```python
from build123d import *

# Parameters (mm, degrees)
BOSS_EXTRUDE1_DEPTH = 6.35
BOSS_EXTRUDE2_DEPTH = 6.604
SKETCH3_W           = 53.34
SKETCH3_H           = 69.85
BOSS_EXTRUDE3_DEPTH = 38.185673152
FILLET1_R           = 2.54
SKETCH4_W           = 25.4
SKETCH4_H           = 25.4
CUT_EXTRUDE1_DEPTH  = 70.358
CUT_EXTRUDE2_DEPTH  = 89.255701154


with BuildPart() as part:
    # Sketch1 → Boss-Extrude1 (new body)
    with BuildSketch(Plane(origin=(0, 0, 0), x_dir=(1, 0, 0), z_dir=(0, 1, 0))):
        with BuildLine():
            Line((-12.7, 0), (-12.7, 25.4))
            ThreePointArc((-12.7, 25.4), (0, 38.1), (12.7, 25.4))
            Line((12.7, 25.4), (12.7, 0))
            ThreePointArc((12.7, 0), (0, -12.7), (-12.7, 0))
        make_face()
    extrude(amount=BOSS_EXTRUDE1_DEPTH)

    # Sketch2 → Boss-Extrude2 (add)
    with BuildSketch(Plane(origin=(0, 6.35, 0), x_dir=(1, 0, 0), z_dir=(0, 1, 0))):
        with BuildLine():
            Line((-6.35, 0), (-6.35, 25.4))
            ThreePointArc((-6.35, 25.4), (0, 31.75), (6.35, 25.4))
            Line((6.35, 25.4), (6.35, 0))
            ThreePointArc((6.35, 0), (0, -6.35), (-6.35, 0))
        make_face()
    extrude(amount=BOSS_EXTRUDE2_DEPTH)

    # Sketch3 → Boss-Extrude3 (add)
    with BuildSketch(Plane(origin=(0, 12.954, 0), x_dir=(1, 0, 0), z_dir=(0, 1, 0))):
        with Locations((0.81256739, 13.33105678)):
            Rectangle(SKETCH3_W, SKETCH3_H)
    extrude(amount=BOSS_EXTRUDE3_DEPTH)

    # Fillet1
    fillet1_edges = [part.edges().sort_by_distance(p)[0] for p in [
        (-12.7, 0, -12.7),
        (0, 0, -38.1),
        (12.7, 0, -12.7),
        (0, 0, 12.7),
    ]]
    fillet(fillet1_edges, radius=FILLET1_R)

    # Sketch4 → Cut-Extrude1 (cut)
    with BuildSketch(Plane(origin=(0, 0, -48.25605678), x_dir=(-1, 0, 0), z_dir=(0, 0, -1))):
        with Locations((0, 38.439673152)):
            Rectangle(SKETCH4_W, SKETCH4_H)
    extrude(amount=-CUT_EXTRUDE1_DEPTH, mode=Mode.SUBTRACT)

    # Sketch5 → Cut-Extrude2 (cut, through all)
    with BuildSketch(Plane(origin=(27.48256739, 0, 0), x_dir=(0, 0, -1), z_dir=(1, 0, 0))):
        with BuildLine():
            Line((0.277921972, 39.339563333), (-13.692078028, 39.339563333))
            ThreePointArc((-13.692078028, 39.339563333), (-16.867078028, 42.514563333), (-13.692078028, 45.689563333))
            Line((-13.692078028, 45.689563333), (0.277921972, 45.689563333))
            ThreePointArc((0.277921972, 45.689563333), (3.452921972, 42.514563333), (0.277921972, 39.339563333))
        make_face()
        with BuildLine():
            Line((25.4, 45.689563333), (39.37, 45.689563333))
            ThreePointArc((39.37, 45.689563333), (42.545, 42.514563333), (39.37, 39.339563333))
            Line((39.37, 39.339563333), (25.4, 39.339563333))
            ThreePointArc((25.4, 39.339563333), (22.225, 42.514563333), (25.4, 45.689563333))
        make_face()
    extrude(amount=-CUT_EXTRUDE2_DEPTH, mode=Mode.SUBTRACT)


solid = part.part
```
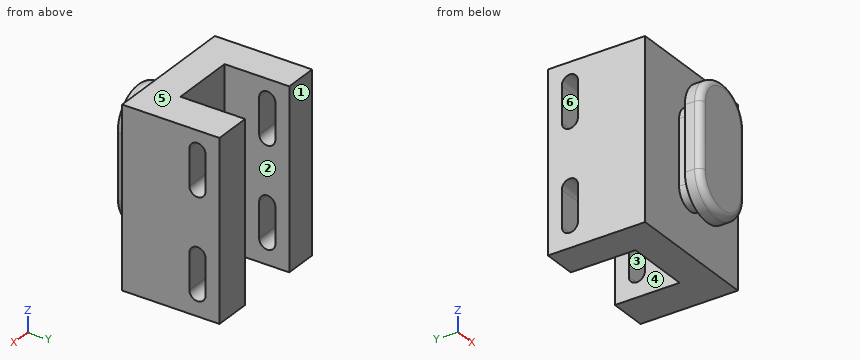
The listing builds one solid part. Answer for the finished solid, in the listing's coordinates (mm). Face numbers are marked on the shaded views. A direction names the side the tool comes from. Coordinates: 2 decimals unless noted, no trailing zeros. Write each loop counter-clockwise with the first axis right and the second up, starting at its lowest first coordinate (ties: lowest second). Pieces come first, ordered by that corner, then holes. Notation, with made-up numbers: M 28.5,58 L 87.5,58 A18 ccw 87.5,77 Z; hole C 33,21.25 d6. An arc over 180 degrees is marked long. Use a Markdown table: item, result. Add a question column.
1. Section C-C (x = 0) is taken. Give the vertices of the cut face in (y, z).
2. Straight lines are drawn through the part: line 1 along Y through (x, z) = (-4.5, -30); line 2 along X through (y, z) = (37, 13.5); line 3 along Y through (x, z) = (-22.5, -26.5). For each, find the intervals that lie inside material, in ascending order. Write a range as [from, to].
3. Given P1, Ø2, axis at x = -13, z = -22.5, coming from the -Y side; P2, Ø8, axis at y = 8, z = -27, coming from the +X side; P3, Ø11, axis at x = 22.5, z = -34, coming from the -Y side, each flat-ended and moving along its own axis, determine where each tip first touches the part or whether it passes through.
4. Section D-D (z = -21) is taken. Give the vertices of the cut face in (x, y).
5. Which of the six approach directions +Z, -Z, +X, -X, +Y, -Y give full straight-line access (tool end or side, diameter ignored) to the marked faces 1, 2 and 3?
6. Section A-A (x = 18) is taken. Give the vertices of the cut face in (y, z) (3 decimals).
7. For a pull along Z with two mould halves and no side action, classify the marked faces 4, 5 and 6 as +Z half, -Z half, draft (parallel to the pull), parting line (faces both ways), or undercut.
8. Section B-B (y = 47) is taken. Give the vertices of the cut face in (x, z), plus the area to 3 significant figures.
Data:
| question | item | result |
|---|---|---|
| 1 | outline | M 0,-35.56 A2.54 ccw 2.54,-38.1 L 6.35,-38.1 L 6.35,-31.75 L 12.95,-31.75 L 12.95,-48.26 L 25.74,-48.26 L 25.74,21.59 L 12.95,21.59 L 12.95,6.35 L 6.35,6.35 L 6.35,12.7 L 2.54,12.7 A2.54 ccw 0,10.16 Z |
| 2 | line 1 | y = [0, 6.35], [12.95, 25.74] |
| 2 | line 2 | x = [-25.86, -12.7], [12.7, 27.48] |
| 2 | line 3 | y = [12.95, 39.34], [45.69, 51.14] |
| 3 | P1 | stops at y = 0.79 |
| 3 | P2 | stops at x = 12.7 |
| 3 | P3 | stops at y = 12.95 |
| 4 | outline | M -25.86,12.95 L -6.35,12.95 L -6.35,6.35 L -12.7,6.35 L -12.7,2.54 A2.54 ccw -10.16,0 L 10.16,0 A2.54 ccw 12.7,2.54 L 12.7,6.35 L 6.35,6.35 L 6.35,12.95 L 27.48,12.95 L 27.48,51.14 L 12.7,51.14 L 12.7,25.74 L -12.7,25.74 L -12.7,51.14 L -25.86,51.14 Z |
| 5 | face 1 | +Z, -Z, +X, -X, +Y |
| 5 | face 2 | +Z, -Z, +Y |
| 5 | face 3 | +X, -X |
| 6 | outline | M 12.954,-48.256 L 51.14,-48.256 L 51.14,21.594 L 12.954,21.594 Z; hole M 39.34,-39.37 A3.175 ccw 45.69,-39.37 L 45.69,-25.4 A3.175 ccw 39.34,-25.4 Z; hole M 39.34,-0.278 A3.175 ccw 45.69,-0.278 L 45.69,13.692 A3.175 ccw 39.34,13.692 Z |
| 7 | face 4 | draft |
| 7 | face 5 | +Z half |
| 7 | face 6 | undercut |
| 8 | outline | M -25.86,-48.26 L -12.7,-48.26 L -12.7,21.59 L -25.86,21.59 Z; M 12.7,-48.26 L 27.48,-48.26 L 27.48,21.59 L 12.7,21.59 Z |
| 8 | area | 1,950 mm2 |
